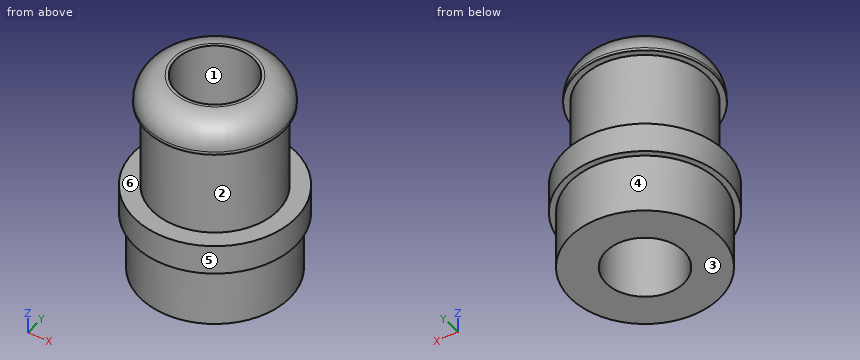
from build123d import *

# Parameters (mm, degrees)
SKETCH1_R           = 2.1
SKETCH1_R_2         = 1.3
BOSS_EXTRUDE1_DEPTH = 7
SKETCH2_R           = 2.5
SKETCH2_R_2         = 2.1
BOSS_EXTRUDE2_DEPTH = 3
BOSS_EXTRUDE3_START = -1
SKETCH3_R           = 2.3
SKETCH3_R_2         = 2.1
BOSS_EXTRUDE3_DEPTH = 1
BOSS_EXTRUDE4_START = -2
SKETCH4_R           = 2.7
SKETCH4_R_2         = 2.5
BOSS_EXTRUDE4_DEPTH = 1
FILLET1_R           = 0.9


with BuildPart() as part:
    # Sketch1 → Boss-Extrude1 (new body)
    with BuildSketch(Plane.XY):
        Circle(SKETCH1_R)
        Circle(SKETCH1_R_2, mode=Mode.SUBTRACT)
    extrude(amount=BOSS_EXTRUDE1_DEPTH)

    # Sketch2 → Boss-Extrude2 (add)
    with BuildSketch(Plane(origin=(0, 0, 0), x_dir=(-1, 0, 0), z_dir=(0, 0, -1))):
        Circle(SKETCH2_R)
        Circle(SKETCH2_R_2, mode=Mode.SUBTRACT)
    extrude(amount=-BOSS_EXTRUDE2_DEPTH)

    # Sketch3 → Boss-Extrude3 (add)
    with BuildSketch(Plane.XY.offset(7).offset(BOSS_EXTRUDE3_START)):
        Circle(SKETCH3_R)
        with Locations(Location((0, 0, 0), (0, 0, 180))):
            Circle(SKETCH3_R_2, mode=Mode.SUBTRACT)
    extrude(amount=BOSS_EXTRUDE3_DEPTH)

    # Sketch4 → Boss-Extrude4 (add)
    with BuildSketch(Plane(origin=(0, 0, 0), x_dir=(-1, 0, 0), z_dir=(0, 0, -1)).offset(BOSS_EXTRUDE4_START)):
        Circle(SKETCH4_R)
        Circle(SKETCH4_R_2, mode=Mode.SUBTRACT)
    extrude(amount=-BOSS_EXTRUDE4_DEPTH)

    # Fillet1
    fillet1_edges = [part.edges().sort_by_distance(p)[0] for p in [
        (-2.3, 0, 7),
    ]]
    fillet(fillet1_edges, radius=FILLET1_R)


solid = part.part
Source: CAD feature listing. Evaluate the final solid. Frame: model axes, mm. Face numbers are marked on the shaded views. A direction names the side the tool comes from. Give positions to 0.01 mm unless a question says otherwise; leave off trailing zeros. Write each loop counter-clockwise with the first axis right and the second up, starting at its lowest first coordinate (ties: lowest second). Pieces come first, ordered by that corner, then holes. Notation, with made-up numbers: M 68,36 L 96,36 A20 ccw 96,62 Z; hole C 80.25,-12 d10. An arc over 180 degrees is marked long. Return JSON: item names as keys, results as strings. Group by question number.
1) Cut plane D-D, the plane z = 1. Output: boundary loops of the cut face in (x, y).
2) Cut plane A-A, the plane x = 0. Output: boundary loops of the cut face in (y, z), then the cut area to 3 significant figures.
3) Cut plane C-C, the plane z = 2.25. Output: boundary loops of the cut face in (x, y), then the cut area to 3 significant figures.
4) First-contact query: pin 1 Ø2 at (y, z) = (2, 0.5) entering from -X; pin 2 Ø3 at (x, z) = (0.5, 5) entering from -Y; pin 3 Ø2 at (x, y) = (0, 0) entering from +Z. Flat tips, straight axial feed; report the tip coordinate or a pass-through.
5) Ray query, L1, parallel to Y at x = 0, z = 4; L2, parallel to X at y = 0.6, z = 2.5; L3, parallel to Z at x = -2.4, y = 0.4. Return the intervals inside material, ascending.
6) Set-up query: the marked faces 4, 5 and 6. Return all of +Z, -Z, +X, -X, +Y, -Y with unobstructed straight access to the full face (end or side cutting, diameter ignored); none if empty.
7) Draft query along X for the marked faces 1, 2 and 3. Return one class per face: released by +X, released by -X, zero draft, split by the parting line, or undercut.
Data:
{
 "1": {"outline": "C 0,0 d5; hole C 0,0 d2.6"},
 "2": {"outline": "M -2.7,2 L -2.5,2 L -2.5,0 L -1.3,0 L -1.3,7 L -1.4,7 A0.9 ccw -2.3,6.1 L -2.3,6 L -2.1,6 L -2.1,3 L -2.7,3 Z; M 1.3,0 L 2.5,0 L 2.5,2 L 2.7,2 L 2.7,3 L 2.1,3 L 2.1,6 L 2.3,6 L 2.3,6.1 A0.9 ccw 1.4,7 L 1.3,7 Z", "area": "14.1 mm²"},
 "3": {"outline": "C 0,0 d5.4; hole C 0,0 d2.6", "area": "17.6 mm²"},
 "4": {"pin 1": "stops at x = -2.29", "pin 2": "stops at y = -2.3", "pin 3": "passes through"},
 "5": {"L1": "y = -2.1 to -1.3, 1.3 to 2.1", "L2": "x = -2.63 to -1.15, 1.15 to 2.63", "L3": "z = 0 to 3"},
 "6": {"face 4": "-Z", "face 5": "+Z, -Z", "face 6": "none"},
 "7": {"face 1": "undercut", "face 2": "split by the parting line", "face 3": "zero draft"}
}
